from build123d import *

# Parameters (mm, degrees)
SKIZZE1_W                       = 45
SKIZZE1_H                       = 65
AUFSATZ_LINEAR_AUSTRAGEN1_DEPTH = 38
SKIZZE2_OUTSIDE_W               = 99.932
SKIZZE2_OUTSIDE_H               = 88.932
SCHNITT_LINEAR_AUSTRAGEN1_DEPTH = 35.4
SCHNITT_LINEAR_AUSTRAGEN2_DEPTH = 25
SKIZZE4_R                       = 1.5
SCHNITT_LINEAR_AUSTRAGEN3_DEPTH = 80.334733881
AUFSATZ_LINEAR_AUSTRAGEN2_DEPTH = 9.6
SKIZZE6_R                       = 16
SCHNITT_LINEAR_AUSTRAGEN4_DEPTH = 7
SKIZZE8_R                       = 13
SCHNITT_LINEAR_AUSTRAGEN5_DEPTH = 185.645606501
SKIZZE9_R                       = 1.5
SCHNITT_LINEAR_AUSTRAGEN6_DEPTH = 185.645606501
SKIZZE12_W                      = 76
SKIZZE12_H                      = 45
AUFSATZ_LINEAR_AUSTRAGEN4_DEPTH = 4
SKIZZE10_W                      = 45
SKIZZE10_H                      = 4
AUFSATZ_LINEAR_AUSTRAGEN3_DEPTH = 15
VERRUNDUNG1_R                   = 15
SKIZZE11_R                      = 2.2
SCHNITT_LINEAR_AUSTRAGEN7_DEPTH = 181.433505758
VERRUNDUNG1_OF_SPIEGELN1_R      = 15
SKIZZE13_R                      = 3.7
SKIZZE13_R_2                    = 1.7
AUFSATZ_LINEAR_AUSTRAGEN5_DEPTH = 9.178687268
SCHNITT_LINEAR_START            = -9.6
SKIZZE14_R                      = 1.7
SCHNITT_LINEAR_AUSTRAGEN8_DEPTH = 9.6
SKIZZE15_R                      = 5
SCHNITT_LINEAR_AUSTRAGEN9_DEPTH = 9.6


with BuildPart() as part:
    # Skizze1 → Aufsatz-Linear austragen1 (new, symmetric)
    with BuildSketch(Plane(origin=(0, 0, 0), x_dir=(0, 0, -1), z_dir=(1, 0, 0))):
        with Locations((0, 32.5)):
            Rectangle(SKIZZE1_W, SKIZZE1_H)
    extrude(amount=AUFSATZ_LINEAR_AUSTRAGEN1_DEPTH, both=True)

    # Skizze2 outside → Schnitt-Linear austragen1 (cut)
    with BuildSketch(Plane.XY.offset(22.5)):
        with Locations((0, 32.5)):
            Rectangle(SKIZZE2_OUTSIDE_W, SKIZZE2_OUTSIDE_H)
        Polygon((-38, 0), (-32, 0), (-23.609003688, 10), (-32, 20), (-32, 45), (-23.609003688, 55), (-32, 65), (-38, 65), align=None, mode=Mode.SUBTRACT)
        Polygon((38, 65), (38, 0), (32, 0), (23.609003688, 10), (32, 20), (32, 45), (23.609003688, 55), (32, 65), align=None, mode=Mode.SUBTRACT)
    extrude(amount=-SCHNITT_LINEAR_AUSTRAGEN1_DEPTH, mode=Mode.SUBTRACT)

    # Skizze3 → Schnitt-Linear austragen2 (cut)
    with BuildSketch(Plane(origin=(0, 0, -22.5), x_dir=(-1, 0, 0), z_dir=(0, 0, -1))):
        with BuildLine():
            Line((-32, 16), (-38, 16))
            Line((-38, 16), (-38, 4))
            Line((-38, 4), (-32, 4))
            ThreePointArc((-32, 4), (-26, 10), (-32, 16))
        make_face()
        with BuildLine():
            Line((38, 16), (38, 4))
            Line((38, 4), (32, 4))
            ThreePointArc((32, 4), (26, 10), (32, 16))
            Line((32, 16), (38, 16))
        make_face()
        with BuildLine():
            Line((32, 49), (38, 49))
            Line((38, 49), (38, 61))
            Line((38, 61), (32, 61))
            ThreePointArc((32, 61), (26, 55), (32, 49))
        make_face()
        with BuildLine():
            Line((-38, 49), (-38, 61))
            Line((-38, 61), (-32, 61))
            ThreePointArc((-32, 61), (-26, 55), (-32, 49))
            Line((-32, 49), (-38, 49))
        make_face()
    extrude(amount=-SCHNITT_LINEAR_AUSTRAGEN2_DEPTH, mode=Mode.SUBTRACT)

    # Skizze4 → Schnitt-Linear austragen3 (cut, through all)
    with BuildSketch(Plane(origin=(0, 0, 2.5), x_dir=(-1, 0, 0), z_dir=(0, 0, -1))):
        with Locations(Location((32, 10, 0), (0, 0, 90))):
            Circle(SKIZZE4_R)
        with Locations(Location((-32, 10, 0), (0, 0, 270))):
            Circle(SKIZZE4_R)
        with Locations(Location((-32, 55, 0), (0, 0, 90))):
            Circle(SKIZZE4_R)
        with Locations(Location((32, 55, 0), (0, 0, 270))):
            Circle(SKIZZE4_R)
    extrude(amount=-SCHNITT_LINEAR_AUSTRAGEN3_DEPTH, mode=Mode.SUBTRACT)

    # Skizze5 → Aufsatz-Linear austragen2 (add)
    with BuildSketch(Plane.XY.offset(-12.9)):
        with BuildLine():
            Line((-38, 65), (38, 65))
            Line((38, 65), (38, 137))
            ThreePointArc((38, 137), (0, 175), (-38, 137))
            Line((-38, 137), (-38, 65))
        make_face()
    extrude(amount=-AUFSATZ_LINEAR_AUSTRAGEN2_DEPTH)

    # Skizze6 → Schnitt-Linear austragen4 (cut)
    with BuildSketch(Plane.XY.offset(-12.9)):
        with Locations((0, 137)):
            Circle(SKIZZE6_R)
    extrude(amount=-SCHNITT_LINEAR_AUSTRAGEN4_DEPTH, mode=Mode.SUBTRACT)

    # Skizze8 → Schnitt-Linear austragen5 (cut, through all)
    with BuildSketch(Plane(origin=(0, 0, -22.5), x_dir=(-1, 0, 0), z_dir=(0, 0, -1))):
        with Locations(Location((0, 137, 0), (0, 0, 90))):
            Circle(SKIZZE8_R)
    extrude(amount=-SCHNITT_LINEAR_AUSTRAGEN5_DEPTH, mode=Mode.SUBTRACT)

    # Skizze9 → Schnitt-Linear austragen6 (cut, through all)
    with BuildSketch(Plane(origin=(0, 0, -22.5), x_dir=(-1, 0, 0), z_dir=(0, 0, -1))):
        with Locations(Location((12.34288865, 70, 0), (0, 0, 90))):
            Circle(SKIZZE9_R)
        with Locations(Location((14.98779336, 85, 0), (0, 0, 90))):
            Circle(SKIZZE9_R)
        with Locations(Location((17.632698071, 100, 0), (0, 0, 90))):
            Circle(SKIZZE9_R)
        with Locations(Location((-12.34288865, 70, 0), (0, 0, 180))):
            Circle(SKIZZE9_R)
        with Locations(Location((-17.632698071, 100, 0), (0, 0, 180))):
            Circle(SKIZZE9_R)
        with Locations(Location((-14.98779336, 85, 0), (0, 0, 180))):
            Circle(SKIZZE9_R)
    extrude(amount=-SCHNITT_LINEAR_AUSTRAGEN6_DEPTH, mode=Mode.SUBTRACT)

    # Skizze12 → Aufsatz-Linear austragen4 (add)
    with BuildSketch(Plane.XZ):
        Rectangle(SKIZZE12_W, SKIZZE12_H)
    extrude(amount=AUFSATZ_LINEAR_AUSTRAGEN4_DEPTH)

    # Skizze10 → Aufsatz-Linear austragen3 (add)
    with BuildSketch(Plane(origin=(38, 0, 0), x_dir=(0, 0, -1), z_dir=(1, 0, 0))):
        with Locations((0, -2)):
            Rectangle(SKIZZE10_W, SKIZZE10_H)
    aufsatz_linear_austragen3 = extrude(amount=AUFSATZ_LINEAR_AUSTRAGEN3_DEPTH)

    # Verrundung1
    verrundung1_edges = [part.edges().sort_by_distance(p)[0] for p in [
        (53, -2, 22.5),
        (53, -2, -22.5),
    ]]
    fillet(verrundung1_edges, radius=VERRUNDUNG1_R)

    # Skizze11 → Schnitt-Linear austragen7 (cut, through all)
    with BuildSketch(Plane(origin=(0, 4, 0), x_dir=(1, 0, 0), z_dir=(0, 1, 0))):
        with Locations(Location((45.5, 10, 0), (0, 0, 180))):
            Circle(SKIZZE11_R)
        with Locations(Location((45.5, -10, 0), (0, 0, 90))):
            Circle(SKIZZE11_R)
    schnitt_linear_austragen7 = extrude(amount=-SCHNITT_LINEAR_AUSTRAGEN7_DEPTH, mode=Mode.SUBTRACT)

    # Spiegeln1: Aufsatz-Linear austragen3, Schnitt-Linear austragen7 across plane
    add(aufsatz_linear_austragen3.mirror(Plane(origin=(0, 0, 0), x_dir=(0, 0, 1), z_dir=(1, 0, 0))))
    add(schnitt_linear_austragen7.mirror(Plane(origin=(0, 0, 0), x_dir=(0, 0, 1), z_dir=(1, 0, 0))), mode=Mode.SUBTRACT)

    # Verrundung1 of Spiegeln1
    verrundung1_of_spiegeln1_edges = [part.edges().sort_by_distance(p)[0] for p in [
        (-53, -2, 22.5),
        (-53, -2, -22.5),
    ]]
    fillet(verrundung1_of_spiegeln1_edges, radius=VERRUNDUNG1_OF_SPIEGELN1_R)

    # Skizze13 → Aufsatz-Linear austragen5 (add)
    # profile 1 of 4: a face of its own
    with BuildSketch(Plane.XY.offset(-12.9)):
        with Locations(Location((-15.5, 36.65, 0), (0, 0, 180))):
            Circle(SKIZZE13_R)
        with Locations(Location((-15.5, 36.65, 0), (0, 0, 180))):
            Circle(SKIZZE13_R_2, mode=Mode.SUBTRACT)
    # profile 2 of 4: a face of its own
    with BuildSketch(Plane.XY.offset(-12.9)):
        with Locations(Location((15.5, 36.65, 0), (0, 0, 180))):
            Circle(SKIZZE13_R)
        with Locations(Location((15.5, 36.65, 0), (0, 0, 180))):
            Circle(SKIZZE13_R_2, mode=Mode.SUBTRACT)
    # profile 3 of 4: a face of its own
    with BuildSketch(Plane.XY.offset(-12.9)):
        with Locations(Location((15.5, 5.65, 0), (0, 0, 180))):
            Circle(SKIZZE13_R)
        with Locations(Location((15.5, 5.65, 0), (0, 0, 180))):
            Circle(SKIZZE13_R_2, mode=Mode.SUBTRACT)
    # profile 4 of 4: a face of its own
    with BuildSketch(Plane.XY.offset(-12.9)):
        with Locations(Location((-15.5, 5.65, 0), (0, 0, 180))):
            Circle(SKIZZE13_R)
        with Locations(Location((-15.5, 5.65, 0), (0, 0, 180))):
            Circle(SKIZZE13_R_2, mode=Mode.SUBTRACT)
    extrude(amount=AUFSATZ_LINEAR_AUSTRAGEN5_DEPTH)

    # Skizze14 → Schnitt-Linear austragen8 (cut)
    with BuildSketch(Plane.XY.offset(-12.9).offset(SCHNITT_LINEAR_START)):
        with Locations(Location((-15.5, 5.65, 0), (0, 0, 180))):
            Circle(SKIZZE14_R)
        with Locations(Location((15.5, 5.65, 0), (0, 0, 180))):
            Circle(SKIZZE14_R)
        with Locations(Location((15.5, 36.65, 0), (0, 0, 180))):
            Circle(SKIZZE14_R)
        with Locations(Location((-15.5, 36.65, 0), (0, 0, 180))):
            Circle(SKIZZE14_R)
    extrude(amount=SCHNITT_LINEAR_AUSTRAGEN8_DEPTH, mode=Mode.SUBTRACT)

    # Skizze15 → Schnitt-Linear austragen9 (cut)
    with BuildSketch(Plane(origin=(0, 0, -22.5), x_dir=(-1, 0, 0), z_dir=(0, 0, -1))):
        with Locations(Location((0, 21.15, 0), (0, 0, 90))):
            Circle(SKIZZE15_R)
    extrude(amount=-SCHNITT_LINEAR_AUSTRAGEN9_DEPTH, mode=Mode.SUBTRACT)


solid = part.part
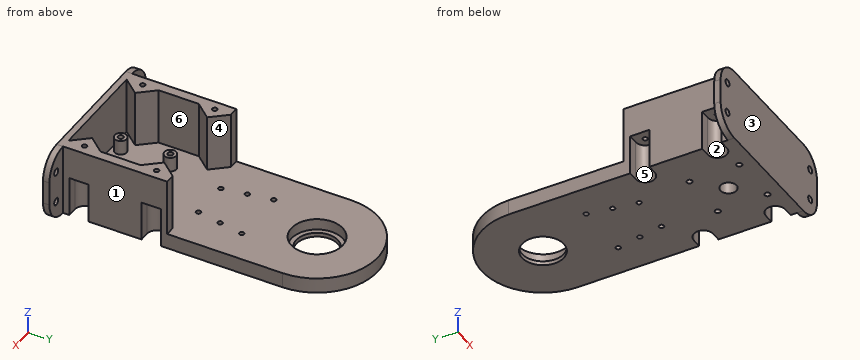
For this review, take the finished solid that the model builds, in its own axes (mm). Face numbers are marked on the shaded views. A direction names the side the tool comes from. Round coordinates to 2 decimals unless told otherwise and drop trailing zeros. Order: outer loops, then holes, each group sorted by start corner. A loop starts at its lowest first (then second) coordinate and runs counter-clockwise, first axis right, second up. Notation, with made-up numbers: (67, -36) -> (74, -36) arc R19 cw to (74, -15) -> close; hole circle Ø5 at (24, 49). An arc over 180 degrees is marked (long way). Write item = value, one per line. Start each with the question number.
1) Take a section at A-A on z = 19.5. State the section outline as (x, y) points, plus the area to 3 significant figures.
2) To check wall thickness, follow line 1 (X direction, y = 55, z = 15.5); line 2 (X direction, y = 31, z = -6); line 3 (X direction, y = 137, z = -21.35). State the ranges of each line that lie inside material, in increasing order. Write a range as from..to.
3) Insertion check: pin 1 (6 mm diameter, centred on x = 17, y = 86.5, fed in from +Z); pin 2 (2.5 mm diameter, centred on x = -45.5, z = -10, fed in from -Y); pin 3 (3.5 mm diameter, centred on x = 16.5, y = 38, fed in from +Z); pin 4 (16 mm diameter, centred on x = -3.5, y = 141, fed in from +Z). Each pin has a flat end and moves straight along its axis. Give the tip position at first contact, or say it passes through.
4) Tool access review of the marked faces 4, 5 and 6: name each direction out of +Z, -Z, +X, -X, +Y, -Y from which nothing blocks a thin tool from reaching the whole face with its end or side.
5) The part is to be moulded in two halves that separate along Y. For the marked faces 1, 2 and 3, say which applies: +Y half, -Y half, draft (parallel to the pull), parting line (faces both ways), or undercut.
6) Take a section at C-C on x = -45.5. State the section outline as (y, z) points, plus the area to 3 significant figures.
7) Take a section at B-B on y = 146. State the section outline as (x, z) points.
8) Take a section at D-D on y = 114. State the section outline as (x, z) points.
Verdict:
q1.outline = (-47, -4) -> (47, -4) -> (47, 0) -> (38, 0) -> (38, 65) -> (32, 65) -> (23.61, 55) -> (32, 45) -> (32, 20) -> (23.61, 10) -> (32, 0) -> (-32, 0) -> (-23.61, 10) -> (-32, 20) -> (-32, 45) -> (-23.61, 55) -> (-32, 65) -> (-38, 65) -> (-38, 0) -> (-47, 0) -> close; hole circle Ø3 at (-32, 10); hole circle Ø3 at (-32, 55); hole circle Ø3 at (32, 10); hole circle Ø3 at (32, 55)
q1.area = 1,460 mm2
q2.line_1 = -38..-33.5, -30.5..-23.61, 23.61..30.5, 33.5..38
q2.line_2 = -38..-32, 32..38
q2.line_3 = -38..-13, 13..38
q3.pin_1 = -12.9
q3.pin_2 = through
q3.pin_3 = -3.72
q3.pin_4 = -19.9
q4.face_4 = +Z, +Y
q4.face_5 = -Z, -X
q4.face_6 = +Z
q5.face_1 = draft
q5.face_2 = undercut
q5.face_3 = -Y half
q6.outline = (-4, -20.49) -> (0, -20.49) -> (0, -12.2) -> (-4, -12.2) -> close; (-4, -7.8) -> (0, -7.8) -> (0, 7.8) -> (-4, 7.8) -> close; (-4, 12.2) -> (0, 12.2) -> (0, 20.49) -> (-4, 20.49) -> close
q6.area = 129 mm2
q7.outline = (-36.92, -22.5) -> (-9.38, -22.5) -> (-9.38, -19.9) -> (-13.23, -19.9) -> (-13.23, -12.9) -> (-36.92, -12.9) -> close; (9.38, -22.5) -> (36.92, -22.5) -> (36.92, -12.9) -> (13.23, -12.9) -> (13.23, -19.9) -> (9.38, -19.9) -> close
q8.outline = (-38, -22.5) -> (38, -22.5) -> (38, -12.9) -> (-38, -12.9) -> close
